Geometry check sheet. Reference: drawing and pictorial views, mm from the part's lowest x, y, z. A direction names the side the tool comes from. Give positions to 0.01 mm unless a question says otherwise; leave off trailing zeros. Order: outer loops, then holes, each group sorted by start corner. A loop starts at its lowest first (then second) coordinate and runs counter-clockwise, first axis right, second up.
Item 1: Sectioned sample at A-A on z = 4. Record the boundary of the cut face in (x, y), and give its area (3 significant figures).
Item 2: Material ranges on line 1 along X through (y, z) = (38, 3); line 2 along Z through (x, y) = (14, 16), recorded low to high.
Item 3: Sectioned sample at B-B on y = 49.5. Record the boundary of the cut face in (x, z), and give its area (3 significant figures).
Item 4: Access from +Z, -Z, +X, -X, +Y, -Y to the whole of each face (thin tool, end or side, straight path). Record for the marked faces 4 and 5.
Item 5: Release check for a two-part mould opening along Y. For the marked faces 1, 2 and 3 record: released by +Y, released by -Y, zero draft, split by the parting line, or undercut.
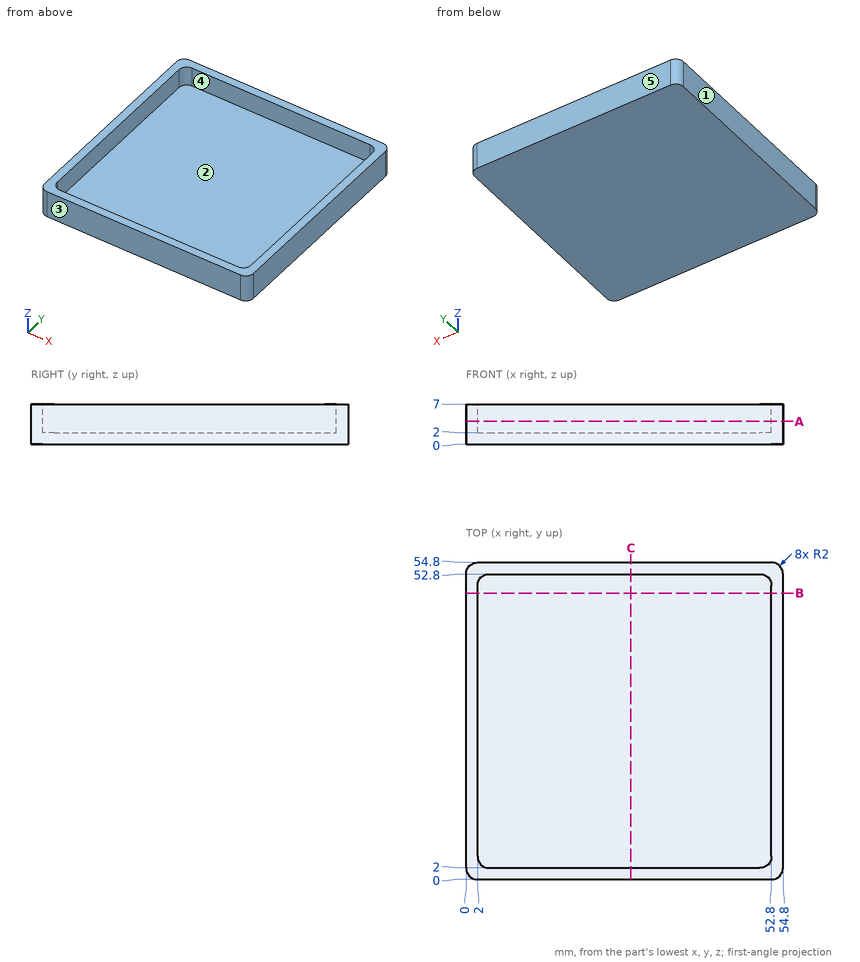
Report:
1. outline: (0, 2) arc R2 ccw to (2, 0) - (52.8, 0) arc R2 ccw to (54.8, 2) - (54.8, 52.8) arc R2 ccw to (52.8, 54.8) - (2, 54.8) arc R2 ccw to (0, 52.8) - close; hole (2, 4) arc R2 ccw to (4, 2) - (50.8, 2) arc R2 ccw to (52.8, 4) - (52.8, 50.8) arc R2 ccw to (50.8, 52.8) - (4, 52.8) arc R2 ccw to (2, 50.8) - close
1. area: 422 mm2
2. line 1: x = 0 to 2, 52.8 to 54.8
2. line 2: z = 0 to 2
3. outline: (0, 0) - (54.8, 0) - (54.8, 7) - (52.8, 7) - (52.8, 2) - (2, 2) - (2, 7) - (0, 7) - close
3. area: 130 mm2
4. face 4: +Z
4. face 5: +Z, -Z, +X, -X, +Y
5. face 1: zero draft
5. face 2: undercut
5. face 3: released by -Y
